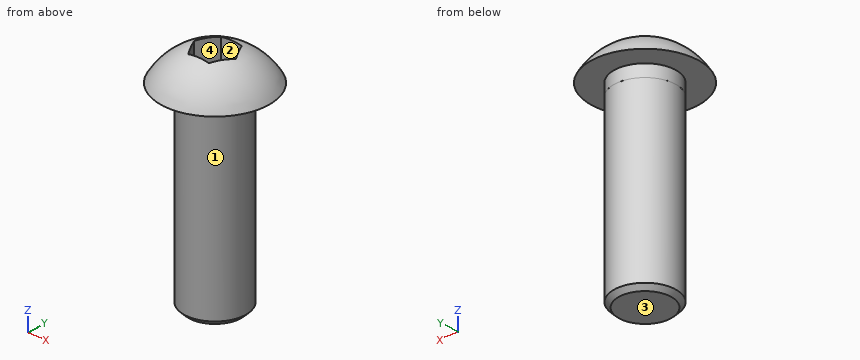
Solid Edge part; units mm, degrees
sketch "Sketch1" plane through (0, 0, 0) normal (1, 0, 0) x (0, 1, 0)
  line L0 (0, -2.1082) -> (0, 2.1082)
  arc A0 (0, 2.1082) -> (6.9469, -2.1082) centre (-0.3606, -6.3169) cw
  line L1 (0, -2.1082) -> (6.9469, -2.1082)
revolve "RevolvedProtrusion1" add sketch "Sketch1" angle 360 about axis through (0, 0, -14.7796) along (0, 0, 1)
sketch "Sketch2" plane through (0, 0, -2.1082) normal (0, 0, -1) x (0, 1, 0)
  circle A0 centre (0, 0) radius 3.9687
extrude "Protrusion1" add sketch "Sketch2" along normal blind 25
sketch "Sketch3" plane through (0, 0, -27.1082) normal (0, 0, -1) x (1, 0, 0)
  circle A0 centre (0, 0) radius 3.9662
extrude "Cutout1" cut sketch "Sketch3" against normal blind 23.4125 flip side to cut
sketch "Sketch4" plane through (-0.6032, 0.3606, 4.2164) normal (0, 0, 1) x (1, 0, 0)
  line L0 (-0.7716, 2.0206) -> (1.978, 2.0206)
  line L1 (3.3529, -0.3606) -> (1.978, 2.0206)
  line L2 (1.978, -2.7419) -> (3.3529, -0.3606)
  line L3 (-0.7716, -2.7419) -> (1.978, -2.7419)
  line L4 (-2.1464, -0.3606) -> (-0.7716, -2.7419)
  line L5 (-0.7716, 2.0206) -> (-2.1464, -0.3606)
extrude "ExtrudedCutout_11" cut sketch "Sketch4" against normal blind 6.3246
chamfer "Chamfer_2" distance 0.6 angle 45 1 edges at (-3.9662, 0, -27.1082)
properties part number "117753"
Verification items for the finished model (mm, model axes). Face numbers are marked on the shaded views. Give positions to 0.01 mm unless a question says otherwise; leave off trailing zeros. Write each loop counter-clockwise with the first axis right and the second up, starting at its lowest first coordinate (ties: lowest second). Pieces come first, ordered by that corner, then holes. Notation, with made-up numbers: (-4.75, 52) - (38.25, 52) arc R29 cw to (38.25, 79) - close; hole circle Ø1 at (-35, 66.5). An arc over 180 degrees is marked (long way). Put each result on its own line as item: value.
Q1. Scan lines: probe 1 along X at (y, z) = (0, -17); probe 2 along X at (y, z) = (-1.5, -20); probe 3 along Y at (x, z) = (-3, -23). Record each from-to range of solid material in increasing order. Write a range as from..to.
Result:
probe 1: -3.97..3.97
probe 2: -3.67..3.67
probe 3: -2.59..2.59
Q2. Section check A-A on z = -4.5. Record the cut outline in (x, y), and give its area (3 significant figures).
Result:
outline: circle Ø7.93 at (0, 0)
area: 49.4 mm2
Q3. Mould release check, pull along X, two halves, no side actions. Record for the marked faces 1, 2, 3 and 4: released by +X, released by -X, zero draft, split by the parting line, or undercut.
Result:
face 1: split by the parting line
face 2: undercut
face 3: zero draft
face 4: undercut
Q4. Depth check by flat-ended pin: P1, Ø1.5, axis at x = 1.5, z = -22, coming from the +Y side; P2, Ø1, axis at x = 4, z = -10.5, coming from the +Y side; P3, Ø1.5, axis at y = 5.5, z = -20.5, coming from the -X side; P4, Ø2, axis at x = 0, z = -0.5, coming from the +Y side. Enter the tip coordinate at first touch or a pass-through.
Result:
P1: y = 3.89
P2: y = 1.87
P3: through
P4: y = 6.56
